For this review, take the finished solid that the model builds, in its own axes (mm). Coordinates: 2 decimals unless noted, no trailing zeros. Write each loop counter-clockwise with the first axis right and the second up, starting at its lowest first coordinate (ties: lowest second). Pieces come first, ordered by that corner, then holes.
1) Insertion check: P1, Ø2.5, axis at x = 0, z = -11.9, coming from the +Y side. The pin has a flat end and moves straight along its axis. Give the tip position at first contact, or say it passes through.
2) We need section B-B on z = 0. Give the number of separate pieces and of enclosed holes in the cut face, then the cut area to 3 significant figures.
3) We need section C-C on z = 5.95. Write out the cut boundary in (x, y).
4) To check wall thickness, follow line 1 along X through (y, z) = (2.4, 0) (3 decimals); line 2 along Z through (x, y) = (0, 2.8); line 3 along Z through (x, y) = (-23.5, 3.8) (3 decimals). State the ranges of each line that lie inside material, in increasing order.
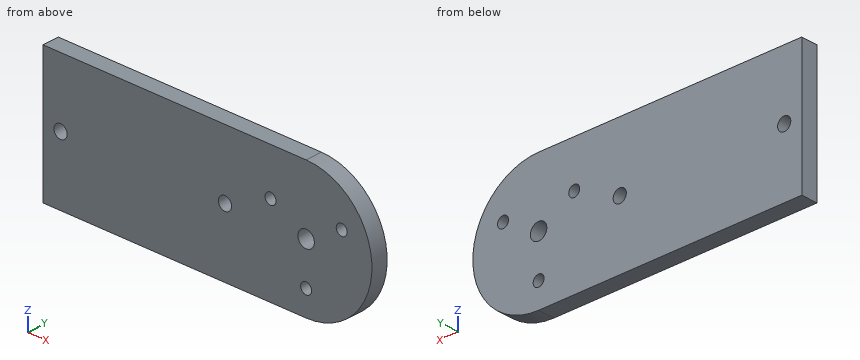
Autodesk Inventor part; units mm, degrees
ref_plane "YZ Plane" through (0, 0, 0) normal (1, 0, 0) x (0, 1, 0)
ref_plane "XZ Plane" through (0, 0, 0) normal (0, 1, 0) x (-1, 0, 0)
ref_plane "XY Plane" through (0, 0, 0) normal (0, 0, 1) x (1, 0, 0)
sketch "Sketch1" plane through (0, 0, 0) normal (0, 1, 0) x (-1, 0, 0)
  circle A0 centre (0, 0) radius 19.05
  dimension "d0" = 38.1
extrude "Extrusion1" add sketch "Sketch1" along normal blind 4.7625
sketch "Sketch2" plane through (0, 4.7625, 0) normal (0, 1, 0) x (1, 0, 0)
  circle A0 centre (0, 0) radius 2.3813
  circle A1 centre (0, 0) radius 19.05
  circle A2 centre (-10.3056, -5.95) radius 1.5875
  circle A3 centre (0, 11.8999) radius 1.5875
  circle A4 centre (10.3056, -5.95) radius 1.5875
  dimension "d3" = 4.7625
  dimension "d4" = 3.175
  dimension "d5" = 3.175
  dimension "d6" = 3.175
extrude "Extrusion2" cut sketch "Sketch2" against normal blind 4.7625 contours A0 | A2 | A3 | A4
sketch "Sketch3" plane through (0, 0, 0) normal (0, -1, 0) x (1, 0, 0)
  circle A0 centre (0, 0) radius 19.05
  line L0 (0, -19.05) -> (0, 19.05)
  line L1 (0, 19.05) -> (-127, 19.05)
  line L2 (-127, 19.05) -> (-127, -19.05)
  line L3 (-127, -19.05) -> (0, -19.05)
  dimension "d9" = 127
extrude "Extrusion3" add sketch "Sketch3" against normal blind 4.7625 contours A0 L3 L2 L1
sketch "Sketch4" plane through (0, 4.7625, 0) normal (0, 1, 0) x (1, 0, 0)
  line L0 (-127, 19.05) -> (-127, -19.05)
  line L1 (-127, 19.05) -> (-76.2, 19.05)
  line L2 (-76.2, 19.05) -> (-76.2, -19.05)
  line L3 (-76.2, -19.05) -> (-127, -19.05)
  line L4 (-127, -19.05) -> (-127, 19.05)
  point P0 (0, 0)
  dimension "d12" = 50.8
extrude "Extrusion4" cut sketch "Sketch4" against normal blind 25.4
sketch "Sketch5" plane through (0, 4.7625, 0) normal (0, 1, 0) x (1, 0, 0)
  line L0 (-76.2, 19.05) -> (-76.2, -19.05)
  line L1 (-76.2, 0) -> (-71.12, 0)
  circle A0 centre (-71.12, 0) radius 1.905
  line L2 (-71.12, 0) -> (-23.495, 0)
  circle A1 centre (-23.495, 0) radius 1.905
  point P0 (0, 0)
  dimension "d15" = 5.08
  dimension "d16" = 3.81
  dimension "d17" = 47.625
  dimension "d18" = 3.81
extrude "Extrusion5" cut sketch "Sketch5" against normal blind 25.4
properties part number "Robotics_PenMount"
Result:
1. P1: passes through
2. separate pieces: 4
2. enclosed holes: 0
2. area: 395 mm2
3. outline: (-76.2, 0) - (-11.89, 0) - (-11.89, 4.76) - (-76.2, 4.76) - close; (-8.72, 0) - (8.72, 0) - (8.72, 4.76) - (-8.72, 4.76) - close; (11.89, 0) - (18.1, 0) - (18.1, 4.76) - (11.89, 4.76) - close
4. line 1: x = -76.2 to -73.025, -69.215 to -25.4, -21.59 to -2.381, 2.381 to 19.05
4. line 2: z = -19.05 to -13.49, -10.31 to -2.38, 2.38 to 19.05
4. line 3: z = -19.05 to -1.905, 1.905 to 19.05
